Autodesk Inventor part; units mm, degrees
ref_plane "YZ Plane" through (0, 0, 0) normal (1, 0, 0) x (0, 1, 0)
ref_plane "XZ Plane" through (0, 0, 0) normal (0, 1, 0) x (-1, 0, 0)
ref_plane "XY Plane" through (0, 0, 0) normal (0, 0, 1) x (1, 0, 0)
sketch "Sketch1" plane through (0, 0, 0) normal (0, 0, 1) x (1, 0, 0)
  line L0 (0, 0) -> (25.4, 0)
  line L1 (25.4, 0) -> (25.4, 25.4)
  line L2 (25.4, 25.4) -> (0, 25.4)
  line L3 (0, 25.4) -> (0, 0)
  dimension "d0" = 25.4
  dimension "d1" = 25.4
extrude "Extrusion1" add sketch "Sketch1" along normal blind 508
shell "Shell1" thickness 2.54 removed faces 2 at (8.4667, 16.9333, 0) at (8.4667, 16.9333, 508)
properties part number "22in"
Input: part model. Units: mm. Frame: model coordinates. A direction names the side the tool comes from. Coordinates: 2 decimals unless noted, no trailing zeros. Loops run counter-clockwise (first coordinate to the right, second up) from the corner with the lowest first, then second, coordinate; pieces in that order, holes last.
(1) First-contact query: pin 1 Ø6 at (x, z) = (5.5, 219.5) entering from -Y. Flat tip, straight axial feed; report the tip coordinate or a pass-through.
(2) Set-up query: faces 5 (the face through (25.4, 13, 250)), 6 (the face through (13, 22.86, 250)). Return all of +Z, -Z, +X, -X, +Y, -Y with unobstructed straight access to the full face (end or side cutting, diameter ignored); none if empty.
(3) Material intervals for probe 1 along Y at (x, z) = (19.75, 81), sorted ascending.
(4) Section A-A on y = 6.5. Return the cut outline in (x, z), then the cut area to 3 significant figures.
(5) Pull-direction query (Y, two-part tool) for faces 1 (the face through (2.54, 13, 250)), 2 (the face through (13, 2.54, 250)), 3 (the face through (13, 0, 250)), 4 (the face through (0, 13, 250)); classes: released by +Y, released by -Y, zero draft, split by the parting line, or undercut.
(6) Section B-B on z = 446. Return the cut outline in (x, y), then the cut area to 3 significant figures.
Data:
1. pin 1: stops at y = 0
2. face 5: +Z, -Z, +X, +Y, -Y
2. face 6: +Z, -Z
3. probe 1: y = 0 to 2.54, 22.86 to 25.4
4. outline: (0, 0) - (2.54, 0) - (2.54, 508) - (0, 508) - close; (22.86, 0) - (25.4, 0) - (25.4, 508) - (22.86, 508) - close
4. area: 2,580 mm2
5. face 1: undercut
5. face 2: undercut
5. face 3: released by -Y
5. face 4: zero draft
6. outline: (0, 0) - (25.4, 0) - (25.4, 25.4) - (0, 25.4) - close; hole (2.54, 2.54) - (22.86, 2.54) - (22.86, 22.86) - (2.54, 22.86) - close
6. area: 232 mm2
